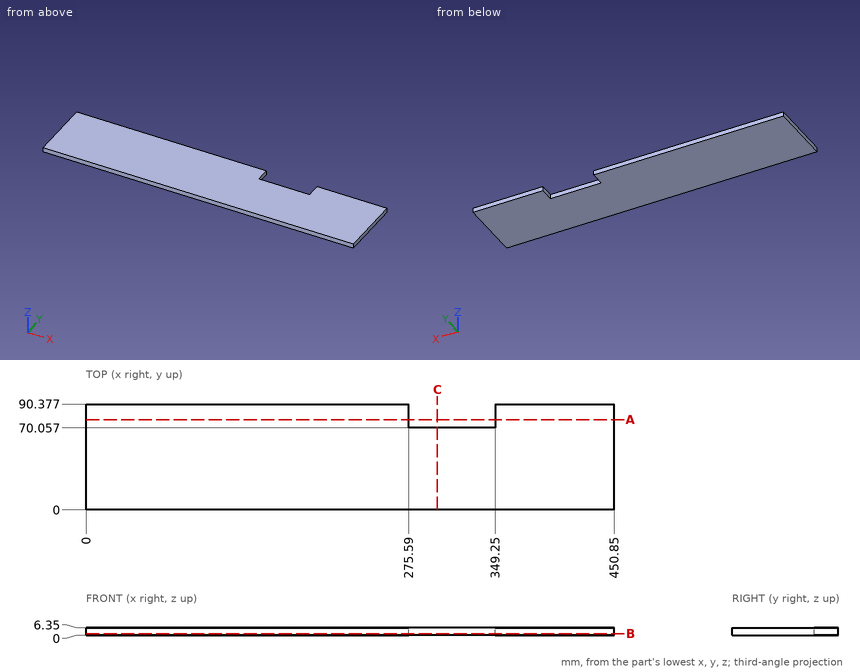
Job drawing, mm, ordinate dimensions from the low corner. One solid piece. Coordinates: 2 decimals unless noted, no trailing zeros. Write each loop counter-clockwise with the first axis right and the second up, starting at its lowest first coordinate (ties: lowest second). Pieces come first, ordered by that corner, then holes. Notation, with made-up numbers: (74.25, 19) -> (111.25, 19) arc R20 ccw to (111.25, 52) -> close; hole circle Ø3 at (15.5, 44.25). An arc over 180 degrees is marked (long way). Use CSV: the item, a comma, the result in double quotes. Start each with the question number.
Item 1: Drop a flat-ended pin along its axis: P1, Ø3, axis at x = 305.5, z = 1, coming from the +Y side. Give the stop position or say it passes through.
Item 2: Band-saw the part on B-B, the plane z = 1.5. Write the cut outline in (x, y), plus the area to 3 significant figures.
Item 3: Band-saw the part on A-A, the plane y = 77. Write the cut outline in (x, z).
Item 4: Wall check: probe 1 along X at (y, z) = (87, 1.5). Give the ranges that are in metal, low to high.
Item 5: Band-saw the part on C-C, the plane x = 300. Write the cut outline in (y, z), plus the area to 3 significant figures.
Response values:
1,P1,"stops at y = 70.06"
2,outline,"(0, 0) -> (450.85, 0) -> (450.85, 90.38) -> (349.25, 90.38) -> (349.25, 70.06) -> (275.59, 70.06) -> (275.59, 90.38) -> (0, 90.38) -> close"
2,area,"39,200 mm2"
3,outline,"(0, 0) -> (275.59, 0) -> (275.59, 6.35) -> (0, 6.35) -> close; (349.25, 0) -> (450.85, 0) -> (450.85, 6.35) -> (349.25, 6.35) -> close"
4,probe 1,"x = 0 to 275.59, 349.25 to 450.85"
5,outline,"(0, 0) -> (70.06, 0) -> (70.06, 6.35) -> (0, 6.35) -> close"
5,area,"445 mm2"
